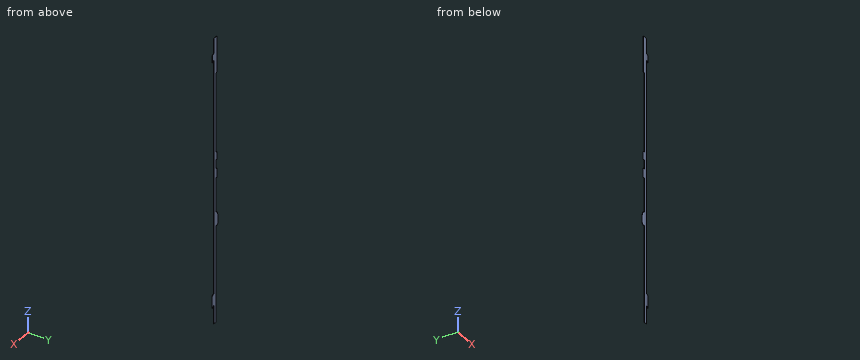
from build123d import *

# Parameters (mm, degrees)
F1_DEPTH = 1270
F2_W     = 1980.1401495934
F2_H     = 3113.6045455933
F3_DEPTH = 299.72


with BuildPart() as f1:
    # F0 (on Top) → F1 (new body, symmetric)
    with BuildSketch(Plane.XY):
        with BuildLine():
            Line((0, -0.7886457275), (0, 0))
            Line((0, 0), (0, 0.6140342441))
            ThreePointArc((0, 0.6140342441), (-18.3170854752, 2.8483369264), (-35.56, 9.4202185041))
            Line((-35.56, 9.4202185041), (-38.1, 9.4202185041))
            ThreePointArc((-38.1, 9.4202185041), (-19.7220112368, 1.8078063092), (0, -0.7886457275))
        make_face()
        with BuildLine():
            Line((0, 0.6140342441), (0, 0))
            Line((0, 0), (0, -0.7886457275))
            ThreePointArc((0, -0.7886457275), (19.7220112368, 1.8078063092), (38.1, 9.4202185041))
            Line((38.1, 9.4202185041), (35.56, 9.4202185041))
            ThreePointArc((35.56, 9.4202185041), (18.3170854752, 2.8483369264), (0, 0.6140342441))
        make_face()
    extrude(amount=F1_DEPTH, both=True)

    # F2 (on Front) → F3 (cut, symmetric)
    with BuildSketch(Plane.XZ):
        with Locations((53.6327660084, 57.6152801514)):
            Rectangle(F2_W, F2_H)
        Polygon((8.1096385542, -557.076325627), (8.1096385542, -654.3815261044), (-8.1096385542, -654.3815261044), (-8.1096385542, -557.076325627), (-8.1096385542, -147.6065518649), (-14.8421686747, -147.6065518649), (-21.5153453208, -136.3835978607), (-21.5153453208, -100.1707464551), (-16.0662650602, -76.3029374071), (-8.1096385542, -76.3029374071), (-8.1096385542, 104.6603173018), (-16.1682730924, 104.6603173018), (-16.1682730924, 151.9920442094), (-8.1096385542, 151.9920442094), (-8.1096385542, 199.323771117), (-16.1682730924, 199.323771117), (-16.1682730924, 240.1269839684), (-9.659161472, 240.1269839684), (-8.1096385542, 240.1269839684), (-8.1096385542, 654.3815261044), (-14.3257157907, 661.1377126473), (-14.3257157907, 847.0746987952), (8.1096385542, 847.0746987952), (8.1096385542, 768.4265060241), (29.4803212851, 768.4265060241), (29.4803212851, 733.0297188755), (8.1096385542, 733.0297188755), (8.1096385542, 654.3815261044), (8.1096385542, -494.1373698037), (36.1618473896, -494.1373698037), (36.1618473896, -557.076325627), align=None, mode=Mode.SUBTRACT)
    extrude(amount=F3_DEPTH, both=True, mode=Mode.SUBTRACT)


solid = f1.part
Design review of the part built by this model. Coordinates are the model's own, in mm. Round coordinates to 2 decimals unless told otherwise and drop trailing zeros. Loops run counter-clockwise (first coordinate to the right, second up) from the corner with the lowest first, then second, coordinate; pieces in that order, holes last. Notation, with made-up numbers: (25.5, 53.5) - (61.5, 53.5) arc R28 cw to (61.5, 80.5) - close; hole circle Ø11 at (-24, 53). An arc over 180 degrees is marked (long way). One line per question, with ' | ' between items.
1. Clearance check with flat-ended pins moving along their axes: P1, Ø0.7, axis at y = 1.5, z = 781, coming from the -X side; P2, Ø0.7, axis at y = 1.5, z = 215, coming from the -X side; P3, Ø0.7, axis at y = 0, z = -1.5, coming from the -X side. State where each tip first meets the part, or that it passes through.
Results are:
P1: stops at x = -14.33 | P2: stops at x = -16.17 | P3: stops at x = -8.11
2. We need section B-B, the plane z = -41.5. State the section outline as (x, y) points.
Results are:
outline: (-8.11, -0.36) arc R76.2 ccw to (8.11, -0.36) - (8.11, 1.05) arc R76.2 cw to (-8.11, 1.05) - close
3. We need section A-A, the plane x = 19. State the section outline as (y, z) points, and give its area (3 significant figures).
Results are:
outline: (1.62, -557.08) - (3.02, -557.08) - (3.02, -494.14) - (1.62, -494.14) - close; (1.62, 733.03) - (3.02, 733.03) - (3.02, 768.43) - (1.62, 768.43) - close | area: 138 mm²
4. For L1, parallel to Z at x = 22, y = 2.5; L2, parallel to Y at x = -15, z = -132.5 (3 decimals); L3, parallel to Y at x = 6.5, z = 35, list the stretches that pass through material, from the lowest coordinate up. Write a range as [from, to].
Results are:
L1: z = [-557.08, -494.14], [733.03, 768.43] | L2: y = [0.702, 2.105] | L3: y = [-0.51, 0.89]
